Check sheet for the modelled part. Datum: model origin and axes. Units: mm. A direction names the side the tool comes from. Round coordinates to 2 decimals unless told otherwise and drop trailing zeros. Write each loop counter-clockwise with the first axis right and the second up, starting at its lowest first coordinate (ties: lowest second). Pieces come first, ordered by that corner, then holes. Notation, with made-up numbers: (74, 50.25) -> (84, 50.25) arc R26 cw to (84, 85.25) -> close; hole circle Ø8 at (77, 46). An arc over 180 degrees is marked (long way). One line per item, written item: value.
Autodesk Inventor part; units mm, degrees
ref_plane "YZ Plane" through (0, 0, 0) normal (1, 0, 0) x (0, 1, 0)
ref_plane "XZ Plane" through (0, 0, 0) normal (0, 1, 0) x (-1, 0, 0)
ref_plane "XY Plane" through (0, 0, 0) normal (0, 0, 1) x (1, 0, 0)
sketch "Sketch1" plane through (0, 0, 0) normal (0, 0, 1) x (1, 0, 0)
  line L0 (0, 0) -> (38.1, 0)
  line L1 (38.1, 0) -> (38.1, 25.4)
  line L2 (38.1, 25.4) -> (0, 25.4)
  line L3 (0, 25.4) -> (0, 0)
  circle A0 centre (6.35, 12.7) radius 2.0701
  line L4 (0, 12.7) -> (38.1, 12.7) construction
  circle A1 centre (31.75, 12.7) radius 2.0701
  dimension "d0" = 38.1
  dimension "d1" = 25.4
  dimension "d2" = 4.1402
  dimension "d3" = 6.35
  dimension "d6" = 25.4
extrude "Plate1" add sketch "Sketch1" along normal blind 3.175
sketch "Sketch2" plane through (0, 26.67, 4.445) normal (0, 1, 0) x (-1, 0, 0)
  line L0 (-38.1, 0) -> (0, 0)
  line L1 (0, 0) -> (0, 40.005)
  line L2 (0, 40.005) -> (-38.1, 40.005)
  line L3 (-38.1, 40.005) -> (-38.1, 0)
edge flange "Flange1" height 44.45 angle 90 thickness 3.175 bend radius 1.27 thickness toward (0, 1, 0) relief tear relief width 3.175 relief depth 1.5875 edges at (19.05, 25.4, 3.175) wall of the first edge with corners at (38.1, 26.67, 4.445) (0, 26.67, 4.445) (0, 26.67, 44.45) (38.1, 26.67, 44.45)
bend "Bend1"
corner "Corner1"
fillet "Fillet1" radius 1.5875 4 edges at (38.1, 0, 1.5875) (0, 0, 1.5875) (38.1, 28.2575, 44.45) (0, 28.2575, 44.45)
sketch "Sketch3" plane through (0, 26.67, 4.445) normal (0, -1, 0) x (1, 0, 0)
  line L0 (0, 38.4175) -> (0, 0)
  line L1 (0, 0) -> (38.1, 0)
  line L2 (9.525, 37.465) -> (28.575, 37.465) construction
  line L3 (28.575, 37.465) -> (28.575, 3.175) construction
  line L4 (28.575, 3.175) -> (9.525, 3.175) construction
  line L5 (9.525, 3.175) -> (9.525, 37.465) construction
  circle A0 centre (25.4, 31.7119) radius 2.413
  line L6 (19.05, 37.465) -> (19.05, 3.175) construction
  line L7 (9.525, 20.32) -> (28.575, 20.32) construction
  circle A1 centre (12.7, 31.7119) radius 2.413
  circle A2 centre (25.4, 8.9281) radius 2.413
  circle A3 centre (12.7, 8.9281) radius 2.413
  point P0 (0, -4.445)
  dimension "d23" = 34.29
  dimension "d24" = 19.05
  dimension "d25" = 3.175
  dimension "d26" = 9.525
  dimension "d27" = 4.826
  dimension "d28" = 3.175
  dimension "d29" = 5.7531
extrude "Extrusion1" cut sketch "Sketch3" against normal blind 25.4
equation "\"d12\" = BendReliefWidth"
equation "\"d13\" = BendReliefDepth"
equation "\"d14\" = MinimumRemnant"
equation "\"d15\" = BendRadius"
equation "\"d19\" = CornerReliefSize"
equation "\"d20\" = GapSize"
equation "\"d21\" = JacobiRadiusSize"
equation "\"BendRadius\" = Thickness"
equation "\"BendReliefWidth\" = Thickness"
equation "\"BendReliefDepth\" = 0.5 * Thickness"
equation "\"CornerReliefSize\" = 4 * Thickness"
equation "\"MinimumRemnant\" = 2 * Thickness"
equation "\"TransitionRadius\" = BendRadius"
equation "\"JacobiRadiusSize\" = BendRadius"
equation "\"GapSize\" = Thickness"
equation "\"d11\" = BendRadius"
properties part number "Pneumatic Piston Back Flange (Custom)" material "Aluminum 6061"
Item 1: Tool access check on faces 5 (the flat face through (19, 13, 3.175)), 6 (the cylindrical face through (37.62, 0.45, 1.61)). Record the directions out of +Z, -Z, +X, -X, +Y, -Y that give a thin tool (end or side, any length) a straight path to the whole face; none if there is none.
Answer:
face 5: +Z, +X, -X, -Y
face 6: +Z, -Z, +X, -Y
Item 2: Sectioned sample at D-D on z = 23. Enter the section's corners in (x, y) (3 decimals), and give its area (3 significant figures).
Answer:
outline: (0, 26.67) -> (38.1, 26.67) -> (38.1, 29.845) -> (0, 29.845) -> close
area: 121 mm^2
Item 3: Sectioned sample at C-C on x = 17.5. Enter the section's corners in (y, z) (3 decimals).
Answer:
outline: (0, 0) -> (25.4, 0) arc R4.445 ccw to (29.845, 4.445) -> (29.845, 44.45) -> (26.67, 44.45) -> (26.67, 4.445) arc R1.27 cw to (25.4, 3.175) -> (0, 3.175) -> close
Item 4: Mould release check, pull along X, two halves, no side actions. Record for faces 1 (the cylindrical face through (18.78, 28.58, 1.34)), 2 (the cylindrical face through (22.99, 28.24, 13.48)), 3 (the cylindrical face through (10.79, 28.24, 11.9)), 4 (the cylindrical face through (37.62, 28.28, 44)): pulls with the +X half, pulls with the -X half, needs draft (parallel to the pull), parting line crosses it, or undercut.
Answer:
face 1: needs draft
face 2: undercut
face 3: undercut
face 4: pulls with the +X half
Item 5: Thickness scan on line 1 (Z direction, x = 25.4, y = 28); line 2 (Z direction, x = 25.4, y = 29); line 3 (Y direction, x = 14.5, z = 40.5) (3 decimals). Record the ranges inside material, lowest first.
Answer:
line 1: z = 0.84 to 10.96, 15.79 to 33.74, 38.57 to 44.45
line 2: z = 1.84 to 10.96, 15.79 to 33.74, 38.57 to 44.45
line 3: y = 26.67 to 29.845
Item 6: Sectioned sample at A-A on x = 25.4. Enter the section's corners in (y, z) (3 decimals).
Answer:
outline: (0, 0) -> (25.4, 0) arc R4.445 ccw to (29.845, 4.445) -> (29.845, 10.96) -> (26.67, 10.96) -> (26.67, 4.445) arc R1.27 cw to (25.4, 3.175) -> (0, 3.175) -> close; (26.67, 15.786) -> (29.845, 15.786) -> (29.845, 33.744) -> (26.67, 33.744) -> close; (26.67, 38.57) -> (29.845, 38.57) -> (29.845, 44.45) -> (26.67, 44.45) -> close
Item 7: Depth check by flat-ended pin: P1, Ø8, axis at x = 5.5, y = 19, coming from the +Z side (3 decimals); P2, Ø5.5, axis at x = 12.7, z = 36.16, coming from the +Y side (3 decimals); P3, Ø6, axis at x = 16.5, z = 25, coming from the -Y side. Enter the tip coordinate at first touch or a pass-through.
Answer:
P1: stops at z = 3.175
P2: stops at y = 29.845
P3: stops at y = 26.67
Item 8: Sectioned sample at B-B on y = 12.7. Enter the section's corners in (x, z) (3 decimals).
Answer:
outline: (0, 0) -> (4.28, 0) -> (4.28, 3.175) -> (0, 3.175) -> close; (8.42, 0) -> (29.68, 0) -> (29.68, 3.175) -> (8.42, 3.175) -> close; (33.82, 0) -> (38.1, 0) -> (38.1, 3.175) -> (33.82, 3.175) -> close
